Input: part model. Units: mm. Frame: model coordinates. Face numbers are marked on the shaded views. A direction names the side the tool comes from. Give positions to 0.01 mm unless a question says otherwise; leave off trailing zeros. Loops run counter-clockwise (first coordinate to the right, second up) from the corner with the lowest first, then second, coordinate; pieces in that order, holes last. Notation, with made-up numbers: M 48,86 L 71,86 A25 ccw 71,107 Z; hole C 62,5 d1. An arc over 180 degrees is marked long. One line per item, written item: value. Start each with the question number.
(1) Ray query, line 1 along Y through (x, z) = (4.5, 1.25); line 2 along Y through (x, z) = (4.25, 0.6); line 3 along X through (y, z) = (-1.5, 0.85). Return the intervals inside material, ascending. Write a range as from..to.
(2) Section B-B on y = 0. Output: boundary loops of the cut face in (x, z).
(3) Pull-direction query (X, two-part tool) for the marked faces 3, 4 and 5; classes: released by +X, released by -X, zero draft, split by the parting line, or undercut.
(4) Section C-C on x = -3.25. State how many separate pieces and enclosed holes the cut face has, plus the area to 3 significant figures.
(5) Access query for the marked faces 1 and 2. Directions: +Z, -Z, +X, -X, +Y, -Y. A direction counts if a zero-diameter tool reaches every point of the face in a straight line with its end or side. Return the directions, or none.
(6) Pin query (flat end, axial travel): P1, Ø1, axis at x = 2.5, y = 2, coming from the +Z side; P2, Ø0.8, axis at x = 3.5, z = 1.5, coming from the -Y side; P3, Ø1.3, axis at x = -4.5, z = 0.5, coming from the +Y side. Return the tip coordinate at first contact, or that it passes through.
```python
from build123d import *

# Parameters (mm, degrees)
F0_R     = 7.62
F1_DEPTH = 2.54
F2_R     = 0.9198153673


# Not quite as in the source:
# - a feature names something its author has since deleted; it is built from what else it names


with BuildPart() as f1:
    # F0 (on Top) → F1 (new body)
    with BuildSketch(Plane.XY):
        Circle(F0_R)
        with BuildLine():
            ThreePointArc((-6.325532194, -0.5569043569), (-6.3438800994, -0.2787207995), (-6.35, 0))
            ThreePointArc((-6.35, 0), (-6.3438800994, 0.2787207995), (-6.325532194, 0.5569043569))
            ThreePointArc((-6.325532194, 0.5569043569), (-4.28871527, 4.6828860047), (0, 6.35))
            ThreePointArc((0, 6.35), (4.28871527, 4.6828860047), (6.325532194, 0.5569043569))
            ThreePointArc((6.325532194, 0.5569043569), (6.3438800994, 0.2787207995), (6.35, 0))
            ThreePointArc((6.35, 0), (6.3438800994, -0.2787207995), (6.325532194, -0.5569043569))
            ThreePointArc((6.325532194, -0.5569043569), (4.28871527, -4.6828860047), (0, -6.35))
            ThreePointArc((0, -6.35), (-4.28871527, -4.6828860047), (-6.325532194, -0.5569043569))
        make_face(mode=Mode.SUBTRACT)
        with BuildLine():
            ThreePointArc((-1.5743877497, 0.5569043569), (-1.6459098023, 0.2825246393), (-1.6699818111, 0))
            Line((-1.6699818111, 0), (0, 0))
            Line((0, 0), (0, 0.5569043569))
            Line((0, 0.5569043569), (-1.5743877497, 0.5569043569))
        make_face()
        with BuildLine():
            ThreePointArc((-6.325532194, 0.5569043569), (-6.3438800994, 0.2787207995), (-6.35, 0))
            Line((-6.35, 0), (-1.6699818111, 0))
            ThreePointArc((-1.6699818111, 0), (-1.6459098023, 0.2825246393), (-1.5743877497, 0.5569043569))
            Line((-1.5743877497, 0.5569043569), (-6.325532194, 0.5569043569))
        make_face()
        with BuildLine():
            Line((-1.6699818111, 0), (-6.35, 0))
            ThreePointArc((-6.35, 0), (-6.3438800994, -0.2787207995), (-6.325532194, -0.5569043569))
            Line((-6.325532194, -0.5569043569), (-1.5743877497, -0.5569043569))
            ThreePointArc((-1.5743877497, -0.5569043569), (-1.6459098023, -0.2825246393), (-1.6699818111, 0))
        make_face()
        with BuildLine():
            Line((0, 0), (-1.6699818111, 0))
            ThreePointArc((-1.6699818111, 0), (-1.6459098023, -0.2825246393), (-1.5743877497, -0.5569043569))
            Line((-1.5743877497, -0.5569043569), (0, -0.5569043569))
            Line((0, -0.5569043569), (0, 0))
        make_face()
        with BuildLine():
            Line((0, 0.5569043569), (0, 0))
            Line((0, 0), (1.6699818111, 0))
            ThreePointArc((1.6699818111, 0), (1.6459098023, 0.2825246393), (1.5743877497, 0.5569043569))
            Line((1.5743877497, 0.5569043569), (0, 0.5569043569))
        make_face()
        with BuildLine():
            Line((1.5743877497, -0.5569043569), (6.325532194, -0.5569043569))
            ThreePointArc((6.325532194, -0.5569043569), (6.3438800994, -0.2787207995), (6.35, 0))
            Line((6.35, 0), (1.6699818111, 0))
            ThreePointArc((1.6699818111, 0), (1.6459098023, -0.2825246393), (1.5743877497, -0.5569043569))
        make_face()
        with BuildLine():
            Line((1.6699818111, 0), (0, 0))
            Line((0, 0), (0, -0.5569043569))
            Line((0, -0.5569043569), (1.5743877497, -0.5569043569))
            ThreePointArc((1.5743877497, -0.5569043569), (1.6459098023, -0.2825246393), (1.6699818111, 0))
        make_face()
        with BuildLine():
            ThreePointArc((1.5743877497, 0.5569043569), (0.9640588941, 1.3636090708), (0, 1.6699818111))
            Line((0, 1.6699818111), (0, 0.5569043569))
            Line((0, 0.5569043569), (1.5743877497, 0.5569043569))
        make_face()
        with BuildLine():
            ThreePointArc((0, 1.6699818111), (-0.9640588941, 1.3636090708), (-1.5743877497, 0.5569043569))
            Line((-1.5743877497, 0.5569043569), (0, 0.5569043569))
            Line((0, 0.5569043569), (0, 1.6699818111))
        make_face()
        with BuildLine():
            Line((0, -0.5569043569), (-1.5743877497, -0.5569043569))
            ThreePointArc((-1.5743877497, -0.5569043569), (-0.9640588941, -1.3636090708), (0, -1.6699818111))
            Line((0, -1.6699818111), (0, -0.5569043569))
        make_face()
        with BuildLine():
            Line((0, -0.5569043569), (0, -1.6699818111))
            ThreePointArc((0, -1.6699818111), (0.9640588941, -1.3636090708), (1.5743877497, -0.5569043569))
            Line((1.5743877497, -0.5569043569), (0, -0.5569043569))
        make_face()
        with BuildLine():
            ThreePointArc((6.35, 0), (6.3438800994, 0.2787207995), (6.325532194, 0.5569043569))
            Line((6.325532194, 0.5569043569), (1.5743877497, 0.5569043569))
            ThreePointArc((1.5743877497, 0.5569043569), (1.6459098023, 0.2825246393), (1.6699818111, 0))
            Line((1.6699818111, 0), (6.35, 0))
        make_face()
    extrude(amount=F1_DEPTH)

    # F2
    f2_edges = [f1.edges().sort_by_distance(p)[0] for p in [
        (-7.62, 0, 2.54),
        (-7.62, 0, 0),
    ]]
    fillet(f2_edges, radius=F2_R)


solid = f1.part
```
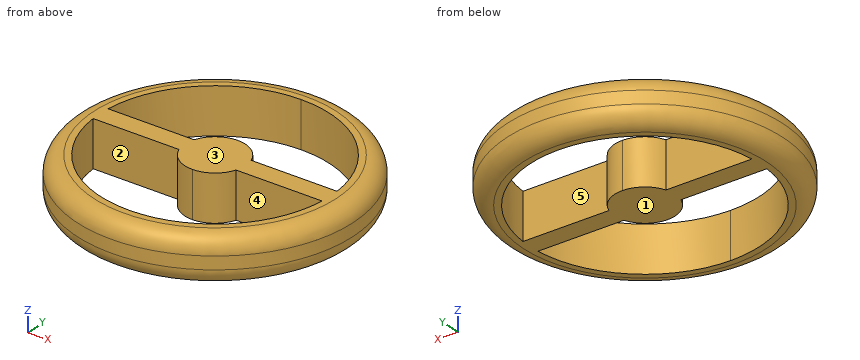
Output values:
1. line 1: y = -6.15..-4.48, -0.56..0.56, 4.48..6.15
1. line 2: y = -6.26..-4.72, -0.56..0.56, 4.72..6.26
1. line 3: x = -7.47..-6.17, -0.73..0.73, 6.17..7.47
2. outline: M -7.62,0.92 A0.92 ccw -6.7,0 L 6.7,0 A0.92 ccw 7.62,0.92 L 7.62,1.62 A0.92 ccw 6.7,2.54 L -6.7,2.54 A0.92 ccw -7.62,1.62 Z
3. face 3: zero draft
3. face 4: undercut
3. face 5: undercut
4. separate pieces: 3
4. enclosed holes: 0
4. area: 9.32 mm²
5. face 1: -Z, +X, -X, +Y, -Y
5. face 2: +Z, -Z
6. P1: passes through
6. P2: stops at y = -6.96
6. P3: stops at y = 6.53
